Can you work these out from the drawing? Everything is in mm from the part's minimum corner. Round coordinates to 2 decimals unless told otherwise and drop trailing zeros. Write each loop counter-clockwise with the first axis right and the second up, starting at its lowest first coordinate (ties: lowest second). Pieces come first, ordered by that corner, then holes. Notation, with made-up numbers: (-28.5, 37.25) -> (9.5, 37.25) arc R17 ccw to (9.5, 66.25) -> close; hole circle Ø11 at (-12.75, 85). An arc over 180 degrees is marked (long way). One line per question, with ' | ' between items. Start each with the question number.
1. If I drill on line 1 along Y through (x, z) = (4, 1.35); line 2 along X through (y, z) = (20, 1.25); line 3 along X through (y, z) = (7, 1), over which ranges is the centre line in solid material (lowest first)? Write a range as [from, to].
2. For pin 1 Ø1 at (x, z) = (3.5, 1.5) entering from +Y; pin 2 Ø0.6 at (x, z) = (36, 1) entering from -Y; pin 3 Ø2 at (x, y) = (4, 8) entering from -Z; pin 4 Ø0.6 at (y, z) = (16, 0.5) entering from +X, each with a flat end and sliding along its axis, tell me the tip position at first contact or that it passes through.
3. Imagine slicing it at A-A, the plane z = 1.1. List the corners of the cut face in (x, y) for me, and give its area (3 significant figures).
4. Imagine slicing it at D-D, the plane y = 2. List the corners of the cut face in (x, z) for me.
5. Imagine slicing it at C-C, the plane x = 4. List the corners of the cut face in (y, z) for me.
6. Imagine slicing it at B-B, the plane y = 8. List the corners of the cut face in (x, z) for me, and give its area (3 significant figures).
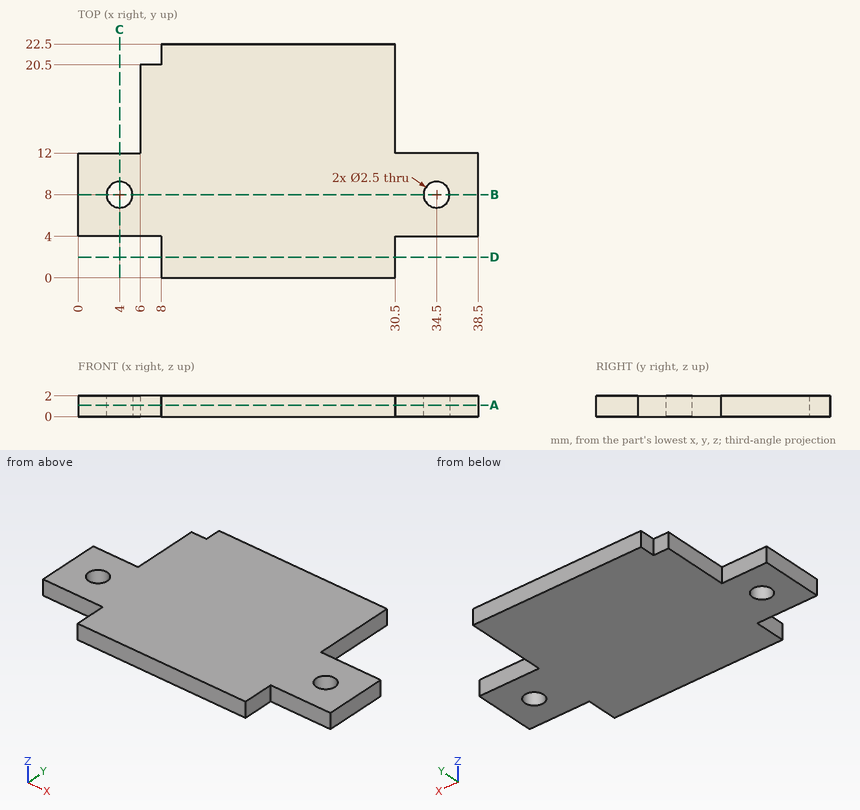
Geometry results:
1) line 1: y = [4, 6.75], [9.25, 12] | line 2: x = [6, 30.5] | line 3: x = [0, 3.25], [4.75, 33.75], [35.25, 38.5]
2) pin 1: stops at y = 12 | pin 2: stops at y = 4 | pin 3: passes through | pin 4: stops at x = 30.5
3) outline: (0, 4) -> (8, 4) -> (8, 0) -> (30.5, 0) -> (30.5, 4) -> (38.5, 4) -> (38.5, 12) -> (30.5, 12) -> (30.5, 22.5) -> (8, 22.5) -> (8, 20.5) -> (6, 20.5) -> (6, 12) -> (0, 12) -> close; hole circle Ø2.5 at (4, 8); hole circle Ø2.5 at (34.5, 8) | area: 641 mm2
4) outline: (8, 0) -> (30.5, 0) -> (30.5, 2) -> (8, 2) -> close
5) outline: (4, 0) -> (6.75, 0) -> (6.75, 2) -> (4, 2) -> close; (9.25, 0) -> (12, 0) -> (12, 2) -> (9.25, 2) -> close
6) outline: (0, 0) -> (2.75, 0) -> (2.75, 2) -> (0, 2) -> close; (5.25, 0) -> (33.25, 0) -> (33.25, 2) -> (5.25, 2) -> close; (35.75, 0) -> (38.5, 0) -> (38.5, 2) -> (35.75, 2) -> close | area: 67.0 mm2
